Input: dimensioned drawing with shaded views. Units: mm. Origin: part minimum x, y, z. Give positions to 0.01 mm unless a question says otherwise; leave off trailing zeros. Order: outer loops, then holes, each group sorted by start corner. A loop starts at its lowest first (then second) coordinate and runs counter-clockwise, first axis right, second up. Notation, with made-up numbers: (-23, 74.25) - (-10, 74.25) arc R21 ccw to (-10, 113.25) - close; hole circle Ø11 at (-12, 5.25). An arc over 180 degrees is marked (long way). Answer as CSV lines item,"result".
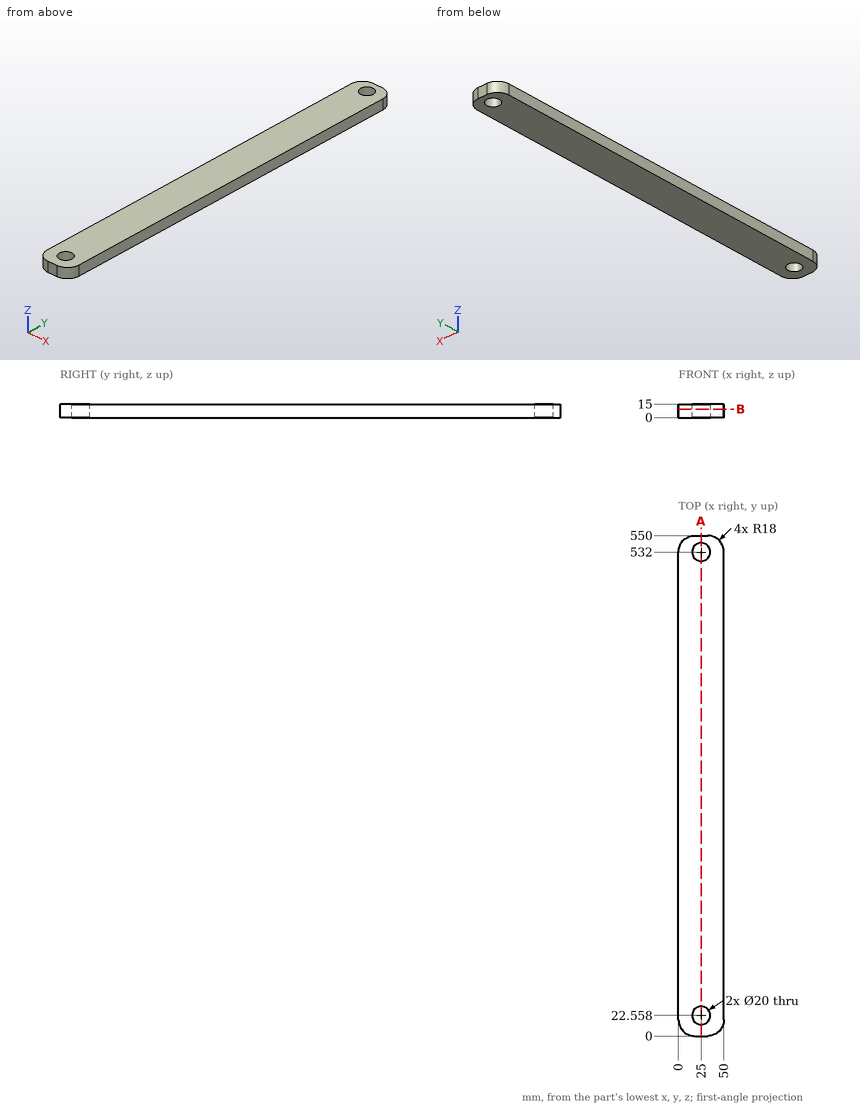
(1) Cut plane B-B (z = 9.5). Return loops of the section in (x, y).
Completed:
outline,"(0, 18) arc R18 ccw to (18, 0) - (32, 0) arc R18 ccw to (50, 18) - (50, 532) arc R18 ccw to (32, 550) - (18, 550) arc R18 ccw to (0, 532) - close; hole circle Ø20 at (25, 22.56); hole circle Ø20 at (25, 532)"
(2) Ray query, line 1 (Y direction, x = 26, z = 8); line 2 (Y direction, x = 25, z = 11); line 3 (X direction, y = 532, z = 8.5). Return the intervals inside material, ascending. Write a range as from..to.
Completed:
line 1,"0..12.61, 32.51..522.05, 541.95..550"
line 2,"0..12.56, 32.56..522, 542..550"
line 3,"0..15, 35..50"
(3) Cut plane A-A (x = 25). Return loops of the section in (y, z), then the cut area to 3 significant figures.
Completed:
outline,"(0, 0) - (12.56, 0) - (12.56, 15) - (0, 15) - close; (32.56, 0) - (522, 0) - (522, 15) - (32.56, 15) - close; (542, 0) - (550, 0) - (550, 15) - (542, 15) - close"
area,"7,650 mm²"
(4) Contact query for flat-ended pins moving along their axis: pin 1 (2 mm diameter, centred on x = 39.5, z = 2, fed in from +Y) (1 decimal); pin 2 (6 mm diameter, centred on x = 36.5, z = 8, fed in from +Y). Output: stop coordinate, or through.
Completed:
pin 1,"y = 548.8"
pin 2,"y = 549.94"
